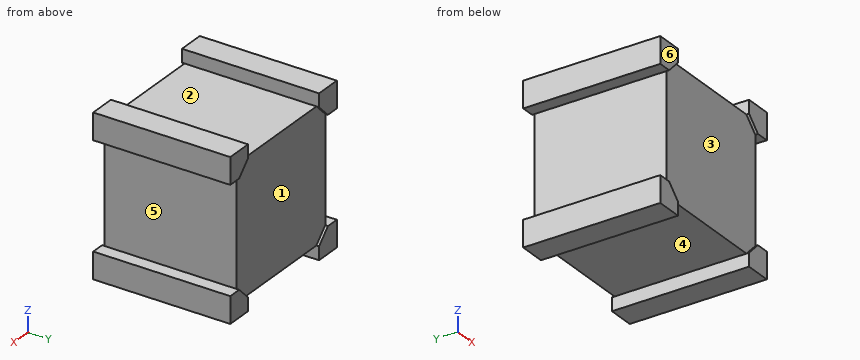
```python
from build123d import *

# Parameters (mm, degrees)
SKETCH1_W           = 12.7
SKETCH1_H           = 12.7
BOSS_EXTRUDE1_DEPTH = 127
BOSS_EXTRUDE2_DEPTH = 2.54


with BuildPart() as part:
    # Sketch1 → Boss-Extrude1 (new body)
    with BuildSketch(Plane(origin=(0, 0, 0), x_dir=(1, 0, 0), z_dir=(0, 1, 0))):
        Polygon((50.8, 63.5), (-50.8, 63.5), (-50.8, 50.8), (-63.5, 50.8), (-63.5, -50.8), (-50.8, -50.8), (-50.8, -63.5), (50.8, -63.5), (50.8, -50.8), (63.5, -50.8), (63.5, 50.8), (50.8, 50.8), align=None)
        with Locations((-57.15, -57.15)):
            Rectangle(SKETCH1_W, SKETCH1_H)
        Polygon((-63.5, -63.5), (-63.5, -50.8), (-76.2, -50.8), (-76.2, -76.2), (-50.8, -76.2), (-50.8, -63.5), align=None)
        with Locations((57.15, -57.15)):
            Rectangle(SKETCH1_W, SKETCH1_H)
        Polygon((76.2, -50.8), (63.5, -50.8), (63.5, -63.5), (50.8, -63.5), (50.8, -76.2), (76.2, -76.2), align=None)
        with Locations((57.15, 57.15)):
            Rectangle(SKETCH1_W, SKETCH1_H)
        Polygon((50.8, 76.2), (50.8, 63.5), (63.5, 63.5), (63.5, 50.8), (76.2, 50.8), (76.2, 76.2), align=None)
        Polygon((-63.5, 50.8), (-63.5, 63.5), (-50.8, 63.5), (-50.8, 76.2), (-76.2, 76.2), (-76.2, 50.8), align=None)
        with Locations((-57.15, 57.15)):
            Rectangle(SKETCH1_W, SKETCH1_H)
    extrude(amount=BOSS_EXTRUDE1_DEPTH)

    # Sketch2 → Boss-Extrude2 (add)
    with BuildSketch(Plane.XZ):
        Polygon((50.8, 63.5), (63.5, 50.8), (76.2, 50.8), (76.2, 76.2), (50.8, 76.2), align=None)
        Polygon((63.5, -50.8), (50.8, -63.5), (50.8, -76.2), (76.2, -76.2), (76.2, -50.8), align=None)
        Polygon((-63.5, -50.8), (-50.8, -63.5), (-50.8, -76.2), (-76.2, -76.2), (-76.2, -50.8), align=None)
        Polygon((-63.5, 50.8), (-50.8, 63.5), (-50.8, 76.2), (-76.2, 76.2), (-76.2, 50.8), align=None)
    boss_extrude2 = extrude(amount=BOSS_EXTRUDE2_DEPTH)

    # Mirror1: Boss-Extrude2 across plane
    add(boss_extrude2.mirror(Plane.ZX.offset(63.5)))


solid = part.part
```
Design review of the part built by this model. Coordinates are the model's own, in mm. Face numbers are marked on the shaded views. A direction names the side the tool comes from. Coordinates: 2 decimals unless noted, no trailing zeros. Loops run counter-clockwise (first coordinate to the right, second up) from the corner with the lowest first, then second, coordinate; pieces in that order, holes last.
Q1. The part is to be moulded in two halves that separate along X. For the marked faces 4, 5 and 6, say which applies: +X half, -X half, draft (parallel to the pull), parting line (faces both ways), or undercut.
Reported:
face 4: undercut
face 5: +X half
face 6: draft
Q2. We need section A-A on z = -59.5. State the section outline as (x, y) points, and give its area (3 significant figures).
Reported:
outline: (-76.2, -2.54) - (-54.8, -2.54) - (-54.8, 0) - (54.8, 0) - (54.8, -2.54) - (76.2, -2.54) - (76.2, 129.54) - (54.8, 129.54) - (54.8, 127) - (-54.8, 127) - (-54.8, 129.54) - (-76.2, 129.54) - close
area: 19,600 mm2
Q3. We need section D-D on z = -32. State the section outline as (x, y) points.
Reported:
outline: (-63.5, 0) - (63.5, 0) - (63.5, 127) - (-63.5, 127) - close
Q4. For pin 1 (12 mm diameter, centred on x = 22.5, y = 106, fed in from -Z); pin 2 (6 mm diameter, centred on y = 74, z = 28, fed in from +X); pin 3 (3 mm diameter, centred on y = 77, z = -24.5, fed in from -X), all flat-tipped, find the tip position at first contact; note any pin that passes through.
Reported:
pin 1: stops at z = -63.5
pin 2: stops at x = 63.5
pin 3: stops at x = -63.5
Q5. Tool access review of the marked faces 1, 2 and 3: name each direction out of +Z, -Z, +X, -X, +Y, -Y from which nothing blocks a thin tool from reaching the whole face with its end or side.
Reported:
face 1: +Y
face 2: +Z, +Y, -Y
face 3: -Y
Q6. We need section B-B on y = 6.5. State the section outline as (x, z) points.
Reported:
outline: (-76.2, -76.2) - (-50.8, -76.2) - (-50.8, -63.5) - (50.8, -63.5) - (50.8, -76.2) - (76.2, -76.2) - (76.2, -50.8) - (63.5, -50.8) - (63.5, 50.8) - (76.2, 50.8) - (76.2, 76.2) - (50.8, 76.2) - (50.8, 63.5) - (-50.8, 63.5) - (-50.8, 76.2) - (-76.2, 76.2) - (-76.2, 50.8) - (-63.5, 50.8) - (-63.5, -50.8) - (-76.2, -50.8) - close
Q7. We need section C-C on x = -42. State the section outline as (y, z) points.
Reported:
outline: (0, -63.5) - (127, -63.5) - (127, 63.5) - (0, 63.5) - close
Q8. To check wall thickness, follow line 1 (Z direction, x = -66.5, y = 92.5); line 2 (Y direction, x = 38.5, z = -17.5); line 3 (Z direction, x = 16, y = 28.5). State the ranges of each line that lie inside material, in increasing order.
Reported:
line 1: z = -76.2 to -50.8, 50.8 to 76.2
line 2: y = 0 to 127
line 3: z = -63.5 to 63.5
